The model under review builds one solid part; all positions refer to its coordinate system, in mm. Coordinates: 2 decimals unless noted, no trailing zeros. Write each loop counter-clockwise with the first axis right and the second up, starting at its lowest first coordinate (ties: lowest second). Pieces come first, ordered by that corner, then holes.
Autodesk Inventor part; units mm, degrees
ref_plane "YZ Plane" through (0, 0, 0) normal (1, 0, 0) x (0, 1, 0)
ref_plane "XZ Plane" through (0, 0, 0) normal (0, 1, 0) x (-1, 0, 0)
ref_plane "XY Plane" through (0, 0, 0) normal (0, 0, 1) x (1, 0, 0)
sketch "Sketch1" plane through (0, 0, 0) normal (0, 1, 0) x (-1, 0, 0)
  line L0 (0, 0) -> (271, 0)
  line L1 (271, 0) -> (271, 84)
  line L2 (271, 84) -> (0, 84)
  line L3 (0, 84) -> (0, 0)
  line L4 (135.5, 84) -> (135.5, 0) construction
  line L5 (0, 84) -> (-6, 84)
  line L6 (-6, 84) -> (-6, 72)
  line L7 (-6, 72) -> (0, 72)
  line L8 (0, 72) -> (0, 84)
  line L9 (0, 0) -> (-6, 0)
  line L10 (-6, 0) -> (-6, 12)
  line L11 (-6, 12) -> (0, 12)
  line L12 (0, 12) -> (0, 0)
  line L13 (271, 84) -> (271, 0)
  line L14 (271, 84) -> (277, 84)
  line L15 (277, 84) -> (277, 72)
  line L16 (277, 72) -> (271, 72)
  line L17 (271, 72) -> (271, 84)
  line L18 (271, 0) -> (277, 0)
  line L19 (277, 0) -> (277, 12)
  line L20 (277, 12) -> (271, 12)
  line L21 (271, 12) -> (271, 0)
  circle A0 centre (194.5, 49.407) radius 4
  circle A1 centre (78.5, 49.407) radius 4
  line L22 (194.5, 49.407) -> (78.5, 49.407) construction
  dimension "d0" = 271
  dimension "d1" = 84
  dimension "d2" = 6
  dimension "d3" = 12
  dimension "d4" = 6
  dimension "d5" = 12
  dimension "d8" = 8
  dimension "d9" = 76.5
  dimension "d10" = 8
  dimension "d11" = 116
  dimension "d13" = 34.593
extrude "Extrusion1" add sketch "Sketch1" along normal blind 3
properties part number "flipper-support"
Item 1: Take a section at B-B, the plane z = 59. Write out the cut boundary in (x, y), plus the area to 3 significant figures.
Solved:
outline: (-271, 0) - (0, 0) - (0, 3) - (-271, 3) - close
area: 813 mm2
Item 2: Take a section at A-A, the plane x = -194.5. Write out the cut boundary in (y, z), plus the area to 3 significant figures.
Solved:
outline: (0, 0) - (3, 0) - (3, 45.41) - (0, 45.41) - close; (0, 53.41) - (3, 53.41) - (3, 84) - (0, 84) - close
area: 228 mm2
Item 3: Mouldability with a two-part tool opening along Z and no side actions: class faces 1 (the face through (-77.63, 1.48, 53.31)), 2 (the face through (-134, 3, 43)) as pulls with the +Z half, pulls with the -Z half, needs draft (parallel to the pull), parting line crosses it, or undercut.
Solved:
face 1: undercut
face 2: needs draft
Item 4: For pin 1 (1.5 mm diameter, centred on y = 2, z = 49.5, fed in from -X), flat-tipped, find the tip position at first contact; note if it passes through.
Solved:
pin 1: stops at x = -271
Item 5: To check wall thickness, follow line 1 along Z through (x, y) = (-194.5, 2); line 2 along X through (y, z) = (0.2, 29). State the ranges of each line that lie inside material, in increasing order.
Solved:
line 1: z = 0 to 45.41, 53.41 to 84
line 2: x = -271 to 0
